Check sheet for the modelled part. Datum: model origin and axes. Units: mm. A direction names the side the tool comes from. Coordinates: 2 decimals unless noted, no trailing zeros. Loops run counter-clockwise (first coordinate to the right, second up) from the corner with the lowest first, then second, coordinate; pieces in that order, holes last. Notation, with made-up numbers: (59, -22.75) - (107, -22.75) arc R25 cw to (107, -4.75) - close; hole circle Ø9 at (-9, 21). An arc over 180 degrees is marked (long way). Use a Markdown table: item, result. Add a question column.
1) Go/stop test with flat-tipped pins: P1, Ø2, axis at x = 12.5, z = -4, coming from the -Y side; P2, Ø25, axis at x = 0, y = 0, coming from the +Z side; P3, Ø8, axis at x = 4.5, z = 2.5, coming from the -Y side; P4, Ø10, axis at x = -2, z = 7.5, coming from the +Y side. Record where each tip stops, or that it passes through.
2) Tool access check on faces 1 (the flat face through (-5, -13, -9)), 2 (the flat face through (5, -13, 9)), 3 (the flat face through (-5, -13, 7)). Record the directions out of +Z, -Z, +X, -X, +Y, -Y that give a thin tool (end or side, any length) a straight path to the whole face; none if there is none.
3) Thickness scan on line 1 (Z direction, x = 11.5, y = 8); line 2 (Y direction, x = 0, z = -8.4); line 3 (Y direction, x = 0, z = -10.05). Record the ranges inside material, lowest first.
4) Sectioned sample at A-A, the plane z = 2.5. Enter the section's corners in (x, y), then the cut area to 3 significant figures.
5) Draft check along X on faces 4 (the flat face through (8, -14, 11)), 5 (the cylindrical face through (-2.799, -21.317, -0.14)), 6 (the cylindrical face through (-2.018, -15.368, 6.014)). Enter one of: pulls with the +X half, pulls with the -X half, needs draft (parallel to the pull), parting line crosses it, or undercut.
6) Sectioned sample at B-B, the plane y = -14.5. State how many separate pieces and enclosed holes the cut face has, then the cut area to 3 significant figures.
from build123d import *


with BuildPart() as part:
    # Эскиз1 → Повернуть1 (revolve)
    with BuildSketch(Plane(origin=(0, 0, 0), x_dir=(0, 0, -1), z_dir=(1, 0, 0)), mode=Mode.PRIVATE) as revolve_1_sk:
        with BuildLine():
            Line((-10, 21.5), (10, 21.5))
            ThreePointArc((10, 21.5), (10.707106781, 21.207106781), (11, 20.5))
            Line((11, 20.5), (11, 15.5))
            Line((11, 15.5), (9, 15.5))
            Line((9, 15.5), (9, 13.5))
            Line((9, 13.5), (7, 13.5))
            Line((7, 13.5), (7, 15.5))
            Line((7, 15.5), (5, 15.5))
            Line((5, 15.5), (5, 13.5))
            Line((5, 13.5), (-5, 13.5))
            Line((-5, 13.5), (-5, 15.5))
            Line((-5, 15.5), (-7, 15.5))
            Line((-7, 15.5), (-7, 13.5))
            Line((-7, 13.5), (-9, 13.5))
            Line((-9, 13.5), (-9, 15.5))
            Line((-9, 15.5), (-11, 15.5))
            Line((-11, 15.5), (-11, 20.5))
            ThreePointArc((-11, 20.5), (-10.707106781, 21.207106781), (-10, 21.5))
        make_face()
    revolve(revolve_1_sk.sketch.rotate(Axis((0, 0, 20.390367039), (0, 0, -1)), 90), axis=Axis((0, 0, 20.390367039), (0, 0, -1)))


solid = part.part
Solved:
| question | item | result |
|---|---|---|
| 1 | P1 | stops at y = -18.17 |
| 1 | P2 | passes through |
| 1 | P3 | stops at y = -21.49 |
| 1 | P4 | stops at y = 21.5 |
| 2 | face 1 | -Z |
| 2 | face 2 | +Z |
| 2 | face 3 | none |
| 3 | line 1 | z = -9 to -7, -5 to 5, 7 to 9 |
| 3 | line 2 | y = -21.5 to -13.5, 13.5 to 21.5 |
| 3 | line 3 | y = -21.5 to -15.5, 15.5 to 21.5 |
| 4 | outline | circle Ø43 at (0, 0); hole circle Ø27 at (0, 0) |
| 4 | area | 880 mm2 |
| 5 | face 4 | needs draft |
| 5 | face 5 | parting line crosses it |
| 5 | face 6 | undercut |
| 6 | separate pieces | 1 |
| 6 | enclosed holes | 2 |
| 6 | area | 610 mm2 |
